Solid Edge part; units mm, degrees
sketch "Sketch1" plane through (0, 0, 0) normal (0, -1, 0) x (1, 0, 0)
  line L0 (0, -8) -> (1.5, -8)
  line L1 (1.5, -8) -> (1.5, -0.115)
  arc A0 (1.5, -0.105) -> (1.5, -0.115) centre (1.5038, -0.11) ccw
  line L2 (1.5, -0.105) -> (1.5, 0)
  line L3 (1.5, 0) -> (2.85, 0)
  line L4 (2.85, 0) -> (2.85, 0.165)
  arc A1 (1.27, 1.65) -> (2.85, 0.165) centre (-0.3628, -1.6703) cw
  line L5 (0, 1.65) -> (1.27, 1.65)
  dimension "D1" = 1.5
revolve "RevolvedProtrusion1" add sketch "Sketch1" angle 360 about axis through (0, 0, 5) along (0, 0, -1)
sketch "Sketch2" plane through (0, 0, 0) normal (0, -1, 0) x (1, 0, 0)
  line L0 (0, -0.0566) -> (1.1545, 0.61)
  line L1 (1.1545, 0.61) -> (1.1545, 1.65)
  line L2 (1.1545, 1.65) -> (0, 1.65)
revolve "RevolvedCutout1" cut sketch "Sketch2" angle 360 about axis through (0, 0, 5.3) along (0, 0, -1)
sketch "Sketch3" plane through (0, 0, 0) normal (0, 0, -1) x (0, 1, 0)
  arc A0 (-1, 0.577) -> (-1, -0.577) centre (0, 0) ccw
  line L0 (-1, 0.577) -> (-1, -0.577)
extrude "Protrusion1" add sketch "Sketch3" against normal blind 1.65
pattern_circular "Pattern1" count 6 over 360 about axis through (0, 0, 0) along (0, 0, -1) of "Protrusion1"
fillet "Round_1" radius 0.185 1 edges at (-1.27, 0, 1.65)
sketch "Sketch4" plane through (0, 0, 0) normal (0, -1, 0) x (1, 0, 0)
  line L0 (0, 0.9501) -> (1.2122, 1.65)
  line L1 (1.2122, 1.65) -> (0, 1.65)
revolve "RevolvedCutout2" cut sketch "Sketch4" angle 360 about axis through (0, 0, 5.3) along (0, 0, -1)
sketch "Sketch5" plane through (0, 0, 0) normal (0, -1, 0) x (1, 0, 0)
  line L0 (-1.5, 0) -> (-1.5, -0.1)
  line L1 (-1.6, 0) -> (-1.5, 0)
  arc A0 (-1.6, 0) -> (-1.5, -0.1) centre (-1.6, -0.1) cw
revolve "RevolvedProtrusion2" add sketch "Sketch5" angle 360 about axis through (0, 0, -0.5) along (0, 0, 1)
cosmetic_thread "Thread1"
chamfer "Chamfer1" distance 0.3065 angle 45 1 edges at (-1.5, 0, -8)
properties material "Stahl"
Build history of the part. All positions in model axes, mm. A direction names the side the tool comes from. Coordinates: 2 decimals unless noted, no trailing zeros. Order: outer loops, then holes, each group sorted by start corner. A loop starts at its lowest first (then second) coordinate and runs counter-clockwise, first axis right, second up. Notation, with made-up numbers: (3.25, -12) -> (14.25, -12) arc R27 ccw to (14.25, 5) -> close; hole circle Ø9 at (-1.75, 44.5). An arc over 180 degrees is marked (long way). One line per item, written item: value.
(1) Slice it at A-A, the plane z = -6.5. List the corners of the cut face in (x, y).
Checked values:
outline: circle Ø3 at (0, 0)
(2) Probe line 1 (Z direction, x = 0.3, y = -1.8); line 2 (X direction, y = -0.05, z = -1.75); line 3 (X direction, y = -0.75, z = -7.5). List the from-to ranges inside material, lowest first. Write a range as [from, to].
Checked values:
line 1: [0, 1.31]
line 2: [-1.5, 1.5]
line 3: [-1.3, 1.3]
(3) Tool access for faces 1 (the flat face through (0, -1, 1)), 2 (the flat face through (0, 2, 0)): list every direction of +Z, -Z, +X, -X, +Y, -Y with a clear straight run to the whole face (end or side of a thin tool).
Checked values:
face 1: +Z
face 2: -Z
(4) Drop flat-ended pins along their axis: pin 1 Ø0.9 at (x, z) = (0, 1) entering from -Y; pin 2 Ø1.2 at (x, z) = (0.5, 1) entering from +Y; pin 3 Ø1.5 at (y, z) = (1, -1.5) entering from -X. Give the stop position or say it passes through.
Checked values:
pin 1: y = -2.6
pin 2: y = 2.67
pin 3: x = -1.48
(5) Mould opens along X. For faces 3 (the cylindrical face through (-1.5, 0.07, -3.85)), 4 (the flat face through (0, 0, -8)), 5 (the flat face through (0.86, 0.51, 1.06)) say: pulls with the +X half, pulls with the -X half, needs draft (parallel to the pull), parting line crosses it, or undercut.
Checked values:
face 3: parting line crosses it
face 4: needs draft
face 5: undercut
